The listing builds one solid part. Answer for the finished solid, in the listing's coordinates (mm). A direction names the side the tool comes from. Give positions to 0.01 mm unless a question says otherwise; leave off trailing zeros. Write each loop counter-clockwise with the first axis right and the second up, starting at its lowest first coordinate (ties: lowest second). Pieces come first, ordered by that corner, then holes. Notation, with made-up numbers: (40, 71) - (91, 71) arc R9 ccw to (91, 79) - close; hole circle Ø1 at (79, 23). An arc over 180 degrees is marked (long way). One line per item, written item: value. Start each with the question number.
from build123d import *

# Parameters (mm, degrees)
PAD006_DEPTH    = 40.5
CHAMFER017_SIZE = 8
THICKNESS_T     = 1
POCKET015_DEPTH = 83.001


with BuildPart() as part:
    # Sketch022 → Pad006 (new body, symmetric)
    with BuildSketch(Plane.YZ):
        with BuildLine():
            ThreePointArc((-21.698485, 29.698485), (-30.80294, 16.072704), (-34, 0))
            Line((-34, 0), (-34, -31.5))
            Line((58, -31.5), (-34, -31.5))
            Line((58, 42), (58, -31.5))
            Line((-9.39697, 42), (58, 42))
            Line((-9.39697, 42), (-21.698485, 29.698485))
        make_face()
    extrude(amount=PAD006_DEPTH, both=True)

    # Chamfer017
    chamfer017_edges = [part.edges().sort_by_distance(p)[0] for p in [
        (-40.5, 58, 5.25),
        (40.5, 58, 5.25),
    ]]
    chamfer(chamfer017_edges, length=CHAMFER017_SIZE)

    # Thickness
    thickness_openings = [part.faces().sort_by_distance(p)[0] for p in [
        (0, 11.624616, -31.5),
    ]]
    offset(amount=THICKNESS_T, openings=thickness_openings)

    # Sketch023 → Pocket015 (cut, through all)
    with BuildSketch(Plane.YZ.offset(41.5)):
        with BuildLine():
            ThreePointArc((34.870058, -26.870058), (8, 38), (-18.870058, -26.870058))
            Line((-8.240115, -37.5), (-18.870058, -26.870058))
            Line((24.240115, -37.5), (-8.240115, -37.5))
            Line((34.870058, -26.870058), (24.240115, -37.5))
        make_face()
    extrude(amount=-POCKET015_DEPTH, mode=Mode.SUBTRACT)


solid = part.part
Item 1: Each of these flat-tipped pins is pushed along its axis until it touches: pin 1 Ø3 at (x, y) = (-6, 32) entering from -Z; pin 2 Ø3 at (x, y) = (1.5, -25) entering from +Z. Where does it stop, or does it pass through?
Item 2: Find section D-D on z = -4.5. Determine the outline of the cut face in (x, y), plus the area to 3 significant figures.
Item 3: The mould has two halves that part along X. Classify faces 4 (the flat face through (1, 24, 42)), 5 (the flat face through (-37.263, 54.651, 5.764)), 6 (the flat face through (41.01, -16.52, -29.22)): +X half, -X half, draft (parallel to the pull), parting line (faces both ways), or undercut.
Item 4: Find section C-C on y = 8. Determine the outline of the cut face in (x, z), plus the area to 3 significant figures.
Item 5: Straight lines are drawn through the part: line 1 along X through (y, z) = (42, 29.5); line 2 along Y through (x, z) = (17.5, -1); line 3 along Z through (x, y) = (-21, 47.5). For each, find the intervals that lie inside material, in ascending order.
Item 6: Find section B-B on y = 42. Determine the outline of the cut face in (x, z), plus the area to 3 significant figures.
Item 7: For faces 1 (the flat face through (-36.6, 53.9, 5.8)), 2 (the flat face through (-40.99, -16.52, -29.22)), 3 (the cylindrical face through (37.05, 54.438, 42.715)), determine the directions among +Z, -Z, +X, -X, +Y, -Y from which every point of the face is accessible in a straight line to the end or side of a thin tool.
Item 8: Find section A-A on x = 6.5. Determine the outline of the cut face in (y, z).
Values:
1. pin 1: z = 42
1. pin 2: z = 29.27
2. outline: (-41.5, -34) arc R1 ccw to (-40.5, -35) - (40.5, -35) arc R1 ccw to (41.5, -34) - (41.5, -29.73) - (40.5, -29.73) - (40.5, -34) - (-40.5, -34) - (-40.5, -29.73) - (-41.5, -29.73) - close; (-41.5, 45.73) - (-40.5, 45.73) - (-40.5, 50) - (-32.5, 58) - (32.5, 58) - (40.5, 50) - (40.5, 45.73) - (41.5, 45.73) - (41.5, 50) arc R1 ccw to (41.21, 50.71) - (33.21, 58.71) arc R1 ccw to (32.5, 59) - (-32.5, 59) arc R1 ccw to (-33.21, 58.71) - (-41.21, 50.71) arc R1 ccw to (-41.5, 50) - close
2. area: 189 mm^2
3. face 4: undercut
3. face 5: -X half
3. face 6: draft
4. outline: (-41.5, 38) - (-40.5, 38) - (-40.5, 42) - (40.5, 42) - (40.5, 38) - (41.5, 38) - (41.5, 42) arc R1 ccw to (40.5, 43) - (-40.5, 43) arc R1 ccw to (-41.5, 42) - close
4. area: 90.6 mm^2
5. line 1: -41.5 to -40.5, 40.5 to 41.5
5. line 2: -35 to -34, 58 to 59
5. line 3: 42 to 43
6. outline: (-41.5, -31.5) - (-40.5, -31.5) - (-40.5, -16.97) - (-41.5, -16.97) - close; (-41.5, 16.97) - (-40.5, 16.97) - (-40.5, 42) - (40.5, 42) - (40.5, 16.97) - (41.5, 16.97) - (41.5, 42) arc R1 ccw to (40.5, 43) - (-40.5, 43) arc R1 ccw to (-41.5, 42) - close; (40.5, -31.5) - (41.5, -31.5) - (41.5, -16.97) - (40.5, -16.97) - close
6. area: 162 mm^2
7. face 1: -Z
7. face 2: +X, -X
7. face 3: +Z, +X, +Y
8. outline: (-35, -31.5) - (-34, -31.5) - (-34, 0) arc R42 cw to (-21.7, 29.7) - (-9.4, 42) - (58, 42) - (58, -31.5) - (59, -31.5) - (59, 42) arc R1 ccw to (58, 43) - (-9.4, 43) arc R1 ccw to (-10.1, 42.71) - (-22.41, 30.41) arc R43 ccw to (-35, 0) - close
